Design review of the part shown in the three views and the two pictorial views. Dimensions are in mm from the part's minimum x, y and z. Give positions to 0.01 mm unless a question says otherwise; leave off trailing zeros. Write each loop counter-clockwise with the first axis right and the second up, starting at its lowest first coordinate (ties: lowest second). Pieces come first, ordered by that corner, then holes. Notation, with made-up numbers: M 63,58 L 88,58 A19 cw 88,92 Z; hole C 35,-2.5 d7. An arc over 180 degrees is marked long. Use one line per item in the form item = value. Start each with the question number.
Q1. Consider section A-A on x = 110. Write out the cut boundary in (y, z), and give its area (3 significant figures).
Q2. For probe 1 along Y at (x, z) = (110, 1.3); probe 2 along X at (y, z) = (153.5, 0.55); probe 3 along Y at (x, z) = (98.5, 1.05), list the stretches that pass through material, from the lowest coordinate up. Write a range as [from, to].
Q3. Consider section C-C on x = 52. Write out the cut boundary in (y, z).
Q4. Clearance check with flat-ended pins moving along their axes: pin 1 Ø1.5 at (x, z) = (50, 1.5) entering from -Y; pin 2 Ø0.9 at (y, z) = (1.5, 2) entering from -X; pin 3 Ø1.5 at (x, z) = (219, 1) entering from -Y; pin 4 Ø6 at (x, y) = (160.5, 144.5) entering from -Z. State where each tip first meets the part, or that it passes through.
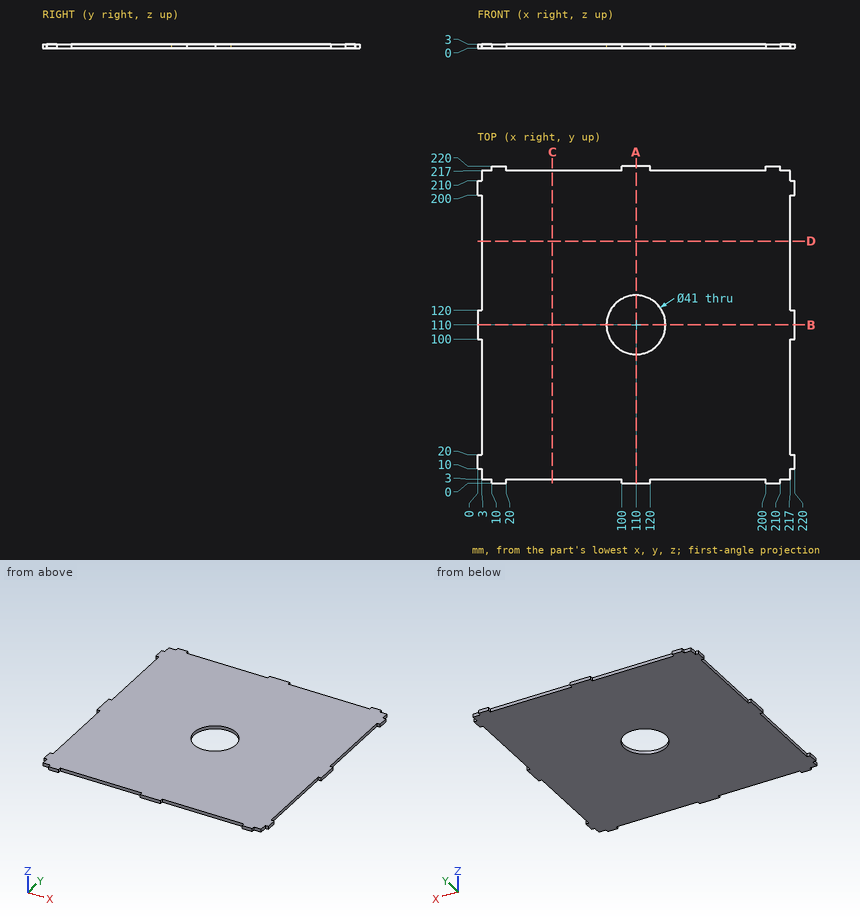
Working result:
q1.outline = M 0,0 L 89.5,0 L 89.5,3 L 0,3 Z; M 130.5,0 L 220,0 L 220,3 L 130.5,3 Z
q1.area = 537 mm²
q2.probe_1 = [0, 89.5], [130.5, 220]
q2.probe_2 = [3, 217]
q2.probe_3 = [3, 93.03], [126.97, 217]
q3.outline = M 3,0 L 217,0 L 217,3 L 3,3 Z
q4.pin_1 = 3
q4.pin_2 = 10
q4.pin_3 = 10
q4.pin_4 = 0
